For this review, use the dimensioned drawing (mm, ordinates from the lowest corner) and the shaded views. A direction names the side the tool comes from. Coordinates: 2 decimals unless noted, no trailing zeros. Write each loop counter-clockwise with the first axis right and the second up, starting at its lowest first coordinate (ties: lowest second). Pieces come first, ordered by that corner, then holes. Notation, with made-up numbers: (85, 16) - (118, 16) arc R24 ccw to (118, 52) - close; hole circle Ø7 at (-22.75, 6). An arc over 180 degrees is marked (long way). Answer as a JSON object with one key per item and string values.
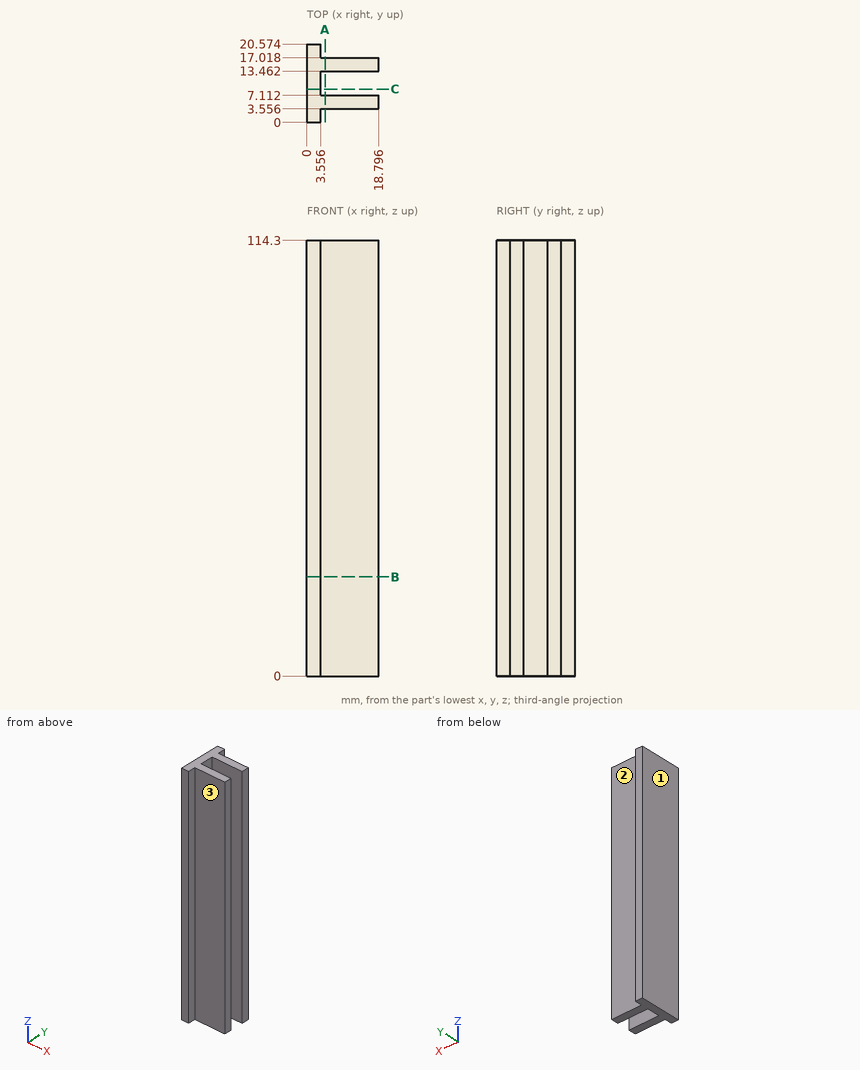
(1) To check wall thickness, follow line 1 (Y direction, x = 11.5, z = 29); line 2 (X direction, y = 8, z = 102). State the ranges of each line that lie inside material, in increasing order. Write a range as from..to.
Solved:
{"line 1": "y = 3.56..7.11, 13.46..17.02", "line 2": "x = 0..3.56"}
(2) Tool access review of the marked faces 1, 2 and 3: name each direction out of +Z, -Z, +X, -X, +Y, -Y from which nothing blocks a thin tool from reaching the whole face with its end or side.
Solved:
{"face 1": "+Z, -Z, -X, +Y, -Y", "face 2": "+Z, -Z, +X, +Y", "face 3": "+Z, -Z, +X, -Y"}
(3) For pin 1 (3 mm diameter, centred on y = 1, z = 46.5, fed in from +X); pin 2 (4.5 mm diameter, centred on x = 13, z = 74.5, fed in from +Y); pin 3 (5 mm diameter, centred on y = 13.5, z = 46.5, fed in from -X); pin 4 (8 mm diameter, centred on x = 12.5, z = 22.5, fed in from -Y), all flat-tipped, find the tip position at first contact; note any pin that passes through.
Solved:
{"pin 1": "stops at x = 3.56", "pin 2": "stops at y = 17.02", "pin 3": "stops at x = 0", "pin 4": "stops at y = 3.56"}
(4) Take a section at A-A, the plane x = 4.75. Write out the cut boundary in (y, z), and give its area (3 significant figures).
Solved:
{"outline": "(3.56, 0) - (7.11, 0) - (7.11, 114.3) - (3.56, 114.3) - close; (13.46, 0) - (17.02, 0) - (17.02, 114.3) - (13.46, 114.3) - close", "area": "813 mm^2"}
(5) Take a section at C-C, the plane y = 8.75. Write out the cut boundary in (x, z).
Solved:
{"outline": "(0, 0) - (3.56, 0) - (3.56, 114.3) - (0, 114.3) - close"}
(6) Take a section at B-B, the plane z = 26. Write out the cut boundary in (x, y).
Solved:
{"outline": "(0, 0) - (3.56, 0) - (3.56, 3.56) - (18.8, 3.56) - (18.8, 7.11) - (3.56, 7.11) - (3.56, 13.46) - (18.8, 13.46) - (18.8, 17.02) - (3.56, 17.02) - (3.56, 20.57) - (0, 20.57) - close"}
